Design review of the part built by this model. Coordinates are the model's own, in mm. A direction names the side the tool comes from. Give positions to 0.01 mm unless a question says otherwise; leave off trailing zeros. Order: outer loops, then holes, each group sorted by start corner. A loop starts at its lowest first (then second) coordinate and runs counter-clockwise, first axis right, second up.
```python
from build123d import *

# Parameters (mm, degrees)
F0_R     = 9.525
F1_DEPTH = 25.4
F2_W     = 12.7
F2_H     = 50.8
F3_DEPTH = 38.1
F4_DEPTH = 25.4
F5_R     = 12.7
F6_DEPTH = 76.2
F7_SIZE2 = 2.54
F7_SIZE  = 2.54


with BuildPart() as f1:
    # F0 (on Front) → F1 (new body, symmetric)
    with BuildSketch(Plane.XZ):
        with BuildLine():
            Line((50.8, 25.4), (0, 25.4))
            ThreePointArc((0, 25.4), (-25.4, 0), (0, -25.4))
            Line((0, -25.4), (50.8, -25.4))
            Line((50.8, -25.4), (50.8, 25.4))
        make_face()
        Circle(F0_R, mode=Mode.SUBTRACT)
    extrude(amount=F1_DEPTH, both=True)

    # F2 (on Right) → F3 (cut)
    with BuildSketch(Plane.YZ):
        with Locations((19.05, 0)):
            Rectangle(F2_W, F2_H)
        with Locations((-19.05, 0)):
            Rectangle(F2_W, F2_H)
    extrude(amount=F3_DEPTH, mode=Mode.SUBTRACT)

    # F2 (on Right) → F4 (cut)
    with BuildSketch(Plane.YZ):
        with Locations((19.05, 0)):
            Rectangle(F2_W, F2_H)
        with Locations((-19.05, 0)):
            Rectangle(F2_W, F2_H)
    extrude(amount=-F4_DEPTH, mode=Mode.SUBTRACT)

    # F5 (on face) → F6 (join)
    with BuildSketch(Plane.YZ.offset(50.8)):
        Circle(F5_R)
    extrude(amount=F6_DEPTH)

    # F7
    f7_edges = [f1.edges().sort_by_distance(p)[0] for p in [
        (127, -12.7, 0),
    ]]
    chamfer(f7_edges, length=F7_SIZE, length2=F7_SIZE2)


solid = f1.part
```
1. For pin 1 (1 mm diameter, centred on x = 69, z = 0, fed in from +Y); pin 2 (8 mm diameter, centred on y = -2.5, z = 11.5, fed in from -X); pin 3 (2 mm diameter, centred on y = 12, z = -13, fed in from -X), all flat-tipped, find the tip position at first contact; note any pin that passes through.
Recorded:
pin 1: stops at y = 12.7
pin 2: stops at x = -24.27
pin 3: stops at x = -22.39
2. Take a section at A-A (y = 0). State the section outline as (x, z) points (3 decimals).
Recorded:
outline: (0, -25.4) - (50.8, -25.4) - (50.8, -12.7) - (124.46, -12.7) - (127, -10.16) - (127, 10.16) - (124.46, 12.7) - (50.8, 12.7) - (50.8, 25.4) - (0, 25.4) arc R25.4 ccw to start; hole circle Ø19.05 at (0, 0)
3. For line 1 along Z through (x, y) = (0, -6) (3 decimals); line 2 along X through (y, z) = (-5.5, 0) (3 decimals); line 3 along X through (y, z) = (18, -22), list the stretches that pass through material, from the lowest coordinate up.
Recorded:
line 1: z = -25.4 to -9.525, 9.525 to 25.4
line 2: x = -25.4 to -9.525, 9.525 to 127
line 3: x = 38.1 to 50.8
4. Take a section at B-B (x = -4). State the section outline as (y, z) points.
Recorded:
outline: (-12.7, -25.08) - (12.7, -25.08) - (12.7, -8.64) - (-12.7, -8.64) - close; (-12.7, 8.64) - (12.7, 8.64) - (12.7, 25.08) - (-12.7, 25.08) - close
5. Draft analysis for pull direction X (two halves, no side actions). For faces 1 (the face through (31, 0, 25.4)), 2 (the face through (127, 0, 0)), 3 (the face through (-7.559, 0.178, -5.796)), state which applies: pulls with the +X half, pulls with the -X half, needs draft (parallel to the pull), parting line crosses it, or undercut.
Recorded:
face 1: needs draft
face 2: pulls with the +X half
face 3: undercut
6. Take a section at D-D (y = -20). State the section outline as (x, z) points, then the cut area to 3 significant figures.
Recorded:
outline: (38.1, -25.4) - (50.8, -25.4) - (50.8, 25.4) - (38.1, 25.4) - close
area: 645 mm2
7. Machinability: for faces 4 (the face through (44, 25.4, 0)), 5 (the face through (13, 12.7, 0)), 6 (the face through (38.1, -19, 0)), 7 (the face through (-25.394, -0.178, 0.559)), 8 (the face through (87.11, -2.75, -12.4)), which of the approach directions +Z, -Z, +X, -X, +Y, -Y give a long, thin tool a straight path to every point of the face, cutting with its end or side? Answer none if there is none.
Recorded:
face 4: +Z, -Z, +X, -X, +Y
face 5: +Z, -Z, -X, +Y
face 6: +Z, -Z, -X, -Y
face 7: -X, +Y, -Y
face 8: +X
8. Take a section at C-C (z = 21). State the section outline as (x, y) points.
Recorded:
outline: (-14.29, -12.7) - (38.1, -12.7) - (38.1, -25.4) - (50.8, -25.4) - (50.8, 25.4) - (38.1, 25.4) - (38.1, 12.7) - (-14.29, 12.7) - close
